The model under review builds one solid part; all positions refer to its coordinate system, in mm. A direction names the side the tool comes from. Round coordinates to 2 decimals unless told otherwise and drop trailing zeros. Write each loop counter-clockwise with the first axis right and the second up, starting at its lowest first coordinate (ties: lowest second). Pieces come first, ordered by that corner, then holes. Notation, with made-up numbers: (18.5, 33.5) -> (22.5, 33.5) arc R26 cw to (22.5, 68.5) -> close; hole circle Ø4 at (86, 8). An arc over 180 degrees is marked (long way). Answer as a JSON object with one key per item and string values. Group by question number.
1) We need section A-A, the plane x = 0. Write out the cut boundary in (y, z), then the cut area to 3 significant figures.
2) Insertion check: pin 1 Ø1 at (x, z) = (-11, 1) entering from -Y; pin 2 Ø6 at (x, y) = (-9.5, 14) entering from +Z; pin 3 Ø1 at (x, z) = (-0.5, 1) entering from +Y; pin 4 Ø1 at (y, z) = (14.5, 0.5) entering from -X. Each pin has a flat end and moves straight along its axis. Give the tip position at first contact, or say it passes through.
3) We need section C-C, the plane y = -3. Write out the cut boundary in (x, z), then the cut area to 3 significant figures.
4) Mouldability with a two-part tool opening along Y and no side actions: class faces 5 (the flat face through (14.1, 3.2, 2)), 6 (the cylindrical face through (4.798, -10.114, 1.493)), 7 (the flat face through (2.288, -17.243, 1.493)) as pulls with the +Y half, pulls with the -Y half, needs draft (parallel to the pull), parting line crosses it, or undercut.
5) Machinability: for faces 1 (the flat face through (1, 0, 0)), 2 (the flat face through (0, 16.529, 1)), 3 (the cylindrical face through (13.9, 2.9, 1.5)), 4 (the cylindrical face through (-4.05, 13.61, 1.49)), which of the approach directions +Z, -Z, +X, -X, +Y, -Y give a long, thin tool a straight path to every point of the face, cutting with its end or side? Answer none if there is none.
6) To check wall thickness, follow probe 1 along Z at (x, y) = (-1, -16); probe 2 along X at (y, z) = (12, 1.6); probe 3 along X at (y, z) = (-13, 1.4). State the ranges of each line that lie inside material, in increasing order. Write a range as [from, to].
7) We need section B-B, the plane z = 0.65. Write out the cut boundary in (x, y), then the cut area to 3 significant figures.
8) We need section D-D, the plane y = -12. Write out the cut boundary in (x, z), then the cut area to 3 significant figures.
from build123d import *

# Parameters (mm, degrees)
RESSALTO_EXTRUS_O1_DEPTH = 1
RESSALTO_EXTRUS_O2_DEPTH = 1
ESBO_O3_W                = 3
ESBO_O3_H                = 3
CORTE_EXTRUS_O1_DEPTH    = 3


with BuildPart() as part:
    # Esboço1 → Ressalto-extrusão1 (new body)
    with BuildSketch(Plane.XY):
        with BuildLine():
            Line((-5.882044961, 17.645439838), (-6.482899016, 19.447931004))
            ThreePointArc((-6.482899016, 19.447931004), (19.9860222, 4.561679146), (2.597250835, -20.334804845))
            Line((2.597250835, -20.334804845), (2.356530026, -18.450115616))
            ThreePointArc((2.356530026, -18.450115616), (-18.133659167, -4.138889372), (-5.882044961, 17.645439838))
        make_face()
    extrude(amount=RESSALTO_EXTRUS_O1_DEPTH)

    # Esboço2 → Ressalto-extrusão2 (add)
    with BuildSketch(Plane.XY.offset(1)):
        with BuildLine():
            Line((-4.490593465, 13.471249769), (-6.482899016, 19.447931004))
            ThreePointArc((-6.482899016, 19.447931004), (19.974805028, 4.610549218), (2.696693068, -20.321856374))
            Line((2.696693068, -20.321856374), (1.867953247, -14.076602952))
            ThreePointArc((1.867953247, -14.076602952), (2.288152222, -14.014433967), (2.706303705, -13.93972454))
            ThreePointArc((2.706303705, -13.93972454), (4.856795522, -10.085239821), (9.211162742, -10.807149529))
            ThreePointArc((9.211162742, -10.807149529), (13.843976353, 3.159797262), (3.60992442, 13.733479009))
            ThreePointArc((3.60992442, 13.733479009), (0, 11.193771705), (-3.60992442, 13.733479009))
            ThreePointArc((-3.60992442, 13.733479009), (-4.052380602, 13.609489757), (-4.490593465, 13.471249769))
        make_face()
    extrude(amount=RESSALTO_EXTRUS_O2_DEPTH)

    # Esboço3 → Corte-extrusão1 (cut, through all)
    with BuildSketch(Plane(origin=(0, 0, 0), x_dir=(-1, 0, 0), z_dir=(0, 0, -1))):
        Polygon((-7.221547804, -11.538551224), (-4.5186412, -12.840202442), (-5.820292417, -15.543109046), (-8.523199021, -14.241457828), align=None)
        with Locations((0, 15.029187597)):
            Rectangle(ESBO_O3_W, ESBO_O3_H)
    extrude(amount=-CORTE_EXTRUS_O1_DEPTH, mode=Mode.SUBTRACT)


solid = part.part
Here are the results:
{
 "1": {"outline": "(-18.6, 0) -> (13.53, 0) -> (13.53, 2) -> (11.19, 2) -> (11.19, 1) -> (-18.6, 1) -> close; (16.53, 0) -> (20.5, 0) -> (20.5, 2) -> (16.53, 2) -> close", "area": "42.4 mm^2"},
 "2": {"pin 1": "stops at y = -15.35", "pin 2": "stops at z = 1", "pin 3": "stops at y = 20.5", "pin 4": "stops at x = -12.25"},
 "3": {"outline": "(-18.36, 0) -> (20.28, 0) -> (20.28, 2) -> (13.88, 2) -> (13.88, 1) -> (-18.36, 1) -> close", "area": "45.0 mm^2"},
 "4": {"face 5": "needs draft", "face 6": "undercut", "face 7": "pulls with the -Y half"},
 "5": {"face 1": "-Z, +X, -X, +Y, -Y", "face 2": "+Z, -Z", "face 3": "+Z", "face 4": "+Z, -Y"},
 "6": {"probe 1": "z = [0, 1]", "probe 2": "x = [-2.35, 2.35], [7.59, 16.62]", "probe 3": "x = [2.72, 4.6], [7.93, 15.85]"},
 "7": {"outline": "(-6.48, 19.45) -> (-5.88, 17.65) arc R18.6 ccw to (2.36, -18.45) -> (2.6, -20.33) arc R20.5 ccw (long way) to start; hole (-1.5, 13.53) -> (1.5, 13.53) -> (1.5, 16.53) -> (-1.5, 16.53) -> close; hole (4.52, -12.84) -> (5.82, -15.54) -> (8.52, -14.24) -> (7.22, -11.54) -> close", "area": "1,190 mm^2"},
 "8": {"outline": "(-14.21, 0) -> (6.26, 0) -> (6.26, 2) -> (3.01, 2) -> (3.01, 1) -> (-14.21, 1) -> close; (7.44, 0) -> (16.62, 0) -> (16.62, 2) -> (7.44, 2) -> close", "area": "42.1 mm^2"}
}
